Can you work these out from the model? Positions are in its coordinate system, mm. Give positions to 0.01 mm unless a question says otherwise; leave off trailing zeros. Loops run counter-clockwise (first coordinate to the right, second up) from the corner with the lowest first, then second, coordinate; pieces in that order, holes last.
from build123d import *

# Parameters (mm, degrees)
SKETCH1_R           = 1.1303
BOSS_EXTRUDE2_DEPTH = 6.35
FILLET1_R           = 1


with BuildPart() as part:
    # Sketch1 → Boss-Extrude2 (new body)
    with BuildSketch(Plane(origin=(0, 0, 0), x_dir=(1, 0, 0), z_dir=(0, 1, 0))):
        with BuildLine():
            Line((-12.7, 50.8), (-101.6, 50.8))
            Line((-101.6, 50.8), (-101.6, 38.1))
            Line((-101.6, 38.1), (-62.7, 38.1))
            ThreePointArc((-62.7, 38.1), (-27.344660941, 23.455339059), (-12.7, -11.9))
            Line((-12.7, -11.9), (-12.7, -50.8))
            Line((-12.7, -50.8), (12.7, -50.8))
            Line((12.7, -50.8), (12.7, 50.8))
            Line((12.7, 50.8), (-12.7, 50.8))
        make_face()
        with Locations(Location((-97.6, 47.7, 0), (0, 0, 270))):
            Circle(SKETCH1_R, mode=Mode.SUBTRACT)
        with Locations(Location((-97.6, 41.2, 0), (0, 0, 270))):
            Circle(SKETCH1_R, mode=Mode.SUBTRACT)
        with Locations(Location((-77.6, 47.7, 0), (0, 0, 270))):
            Circle(SKETCH1_R, mode=Mode.SUBTRACT)
        with Locations(Location((-77.6, 41.2, 0), (0, 0, 270))):
            Circle(SKETCH1_R, mode=Mode.SUBTRACT)
        with BuildLine():
            Line((-3.175, -38.1), (-3.175, 38.1))
            ThreePointArc((-3.175, 38.1), (0, 41.275), (3.175, 38.1))
            Line((3.175, 38.1), (3.175, -38.1))
            ThreePointArc((3.175, -38.1), (0, -41.275), (-3.175, -38.1))
        make_face(mode=Mode.SUBTRACT)
    extrude(amount=BOSS_EXTRUDE2_DEPTH)

    # Fillet1
    fillet1_edges = [part.edges().sort_by_distance(p)[0] for p in [
        (12.7, 3.175, 50.8),
        (-12.7, 3.175, 50.8),
        (-101.6, 3.175, -38.1),
        (-101.6, 3.175, -50.8),
        (12.7, 3.175, -50.8),
    ]]
    fillet(fillet1_edges, radius=FILLET1_R)


solid = part.part
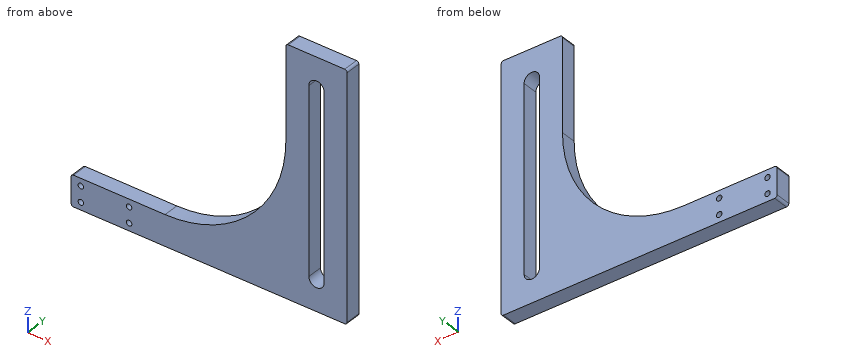
(1) Will these pins go through, and if not, where does the flat tip stop? P1, Ø1.8, axis at x = -77.6, z = -41.2, coming from the +Y side; P2, Ø3, axis at x = -57.5, y = 5, coming from the +Z side; P3, Ø3, axis at x = -53, y = 5.5, coming from the +Z side; P4, Ø1, axis at x = -62, y = 2, coming from the +Z side.
Returned:
P1: passes through
P2: stops at z = -37.65
P3: stops at z = -36.83
P4: stops at z = -38.09
(2) Suppose I cut it at D-D on x = -75. List the corners of the cut face in (y, z) for me.
Returned:
outline: (0, -50.8) - (6.35, -50.8) - (6.35, -38.1) - (0, -38.1) - close
(3) Suppose I cut it at A-A on x = 0. List the corners of the cut face in (y, z) for me (3 decimals), plus the area to 3 significant figures.
Returned:
outline: (0, -50.8) - (6.35, -50.8) - (6.35, -41.275) - (0, -41.275) - close; (0, 41.275) - (6.35, 41.275) - (6.35, 50.8) - (0, 50.8) - close
area: 121 mm2
(4) Suppose I cut it at C-C on z = -10. List the corners of the cut face in (x, y) for me (3 decimals).
Returned:
outline: (-17.751, 0) - (-3.175, 0) - (-3.175, 6.35) - (-17.751, 6.35) - close; (3.175, 0) - (12.7, 0) - (12.7, 6.35) - (3.175, 6.35) - close
(5) Suppose I cut it at B-B on y = 5. List the corners of the cut face in (x, z) for me (3 decimals).
Returned:
outline: (-101.6, -49.8) arc R1 ccw to (-100.6, -50.8) - (11.7, -50.8) arc R1 ccw to (12.7, -49.8) - (12.7, 49.8) arc R1 ccw to (11.7, 50.8) - (-11.7, 50.8) arc R1 ccw to (-12.7, 49.8) - (-12.7, 11.9) arc R50 cw to (-62.7, -38.1) - (-100.6, -38.1) arc R1 ccw to (-101.6, -39.1) - close; hole circle Ø2.261 at (-97.6, -47.7); hole circle Ø2.261 at (-97.6, -41.2); hole circle Ø2.261 at (-77.6, -47.7); hole circle Ø2.261 at (-77.6, -41.2); hole (-3.175, -38.1) arc R3.175 ccw to (3.175, -38.1) - (3.175, 38.1) arc R3.175 ccw to (-3.175, 38.1) - close
(6) Please list where these lines run through material, in increasing order: probe 1 along X at (y, z) = (4.5, -47.7); probe 2 along Z at (x, y) = (-77.6, 1.5); probe 3 along X at (y, z) = (3.5, 20) (3 decimals).
Returned:
probe 1: x = -101.6 to -98.73, -96.47 to -78.73, -76.47 to 12.7
probe 2: z = -50.8 to -48.83, -46.57 to -42.33, -40.07 to -38.1
probe 3: x = -12.7 to -3.175, 3.175 to 12.7
